```python
from build123d import *

# Parameters (mm, degrees)
BOSS_EXTRUDE1_DEPTH = 5


with BuildPart() as part:
    # Sketch1 → Boss-Extrude1 (new body)
    with BuildSketch(Plane(origin=(0, 0, 0), x_dir=(1, 0, 0), z_dir=(0, 1, 0))):
        with BuildLine():
            Line((16.51, -1.905), (16.51, 1.905))
            Line((16.51, 1.905), (12.556312158, 1.905))
            ThreePointArc((12.556312158, 1.905), (8.980256121, 8.980256121), (1.905, 12.556312158))
            Line((1.905, 12.556312158), (1.905, 16.51))
            Line((1.905, 16.51), (-1.905, 16.51))
            Line((-1.905, 16.51), (-1.905, 12.556312158))
            ThreePointArc((-1.905, 12.556312158), (-8.980256121, 8.980256121), (-12.556312158, 1.905))
            Line((-12.556312158, 1.905), (-16.51, 1.905))
            Line((-16.51, 1.905), (-16.51, -1.905))
            Line((-16.51, -1.905), (-12.556312158, -1.905))
            ThreePointArc((-12.556312158, -1.905), (-8.980256121, -8.980256121), (-1.905, -12.556312158))
            Line((-1.905, -12.556312158), (-1.905, -16.51))
            Line((-1.905, -16.51), (1.905, -16.51))
            Line((1.905, -16.51), (1.905, -12.556312158))
            ThreePointArc((1.905, -12.556312158), (8.980256121, -8.980256121), (12.556312158, -1.905))
            Line((12.556312158, -1.905), (16.51, -1.905))
        make_face()
    extrude(amount=BOSS_EXTRUDE1_DEPTH)


solid = part.part
```
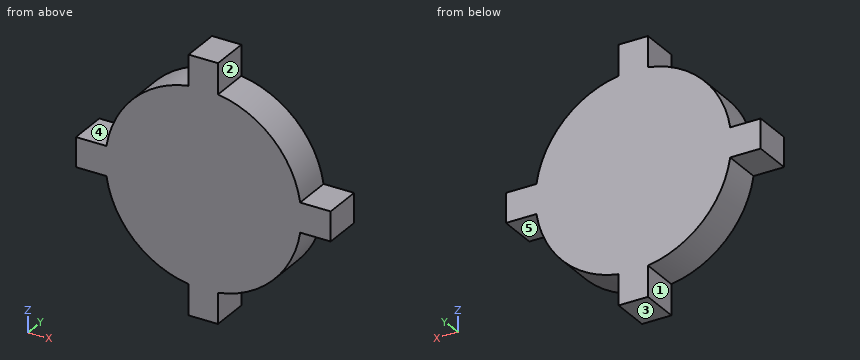
Input: part model. Units: mm. Frame: model coordinates. Face numbers are marked on the shaded views. A direction names the side the tool comes from. Give positions to 0.01 mm unless a question says otherwise; leave off trailing zeros. Loops run counter-clockwise (first coordinate to the right, second up) from the corner with the lowest first, then second, coordinate; pieces in that order, holes last.
1) Section query C-C on x = 14. Return the cut outline in (y, z) (3 decimals), and give its area (4 significant figures).
A:
outline: (0, -1.905) - (5, -1.905) - (5, 1.905) - (0, 1.905) - close
area: 19.05 mm2
2) Line query: L1, parallel to X at y = 0.95, z = 13 (3 decimals); L2, parallel to Z at x = 10.5, y = 3.8. Output: solid intervals per line, ascending.
A:
L1: x = -1.905 to 1.905
L2: z = -7.14 to 7.14
3) Section query A-A on y = 4.2. Return the cut outline in (x, z) (3 decimals).
A:
outline: (-16.51, -1.905) - (-12.556, -1.905) arc R12.7 ccw to (-1.905, -12.556) - (-1.905, -16.51) - (1.905, -16.51) - (1.905, -12.556) arc R12.7 ccw to (12.556, -1.905) - (16.51, -1.905) - (16.51, 1.905) - (12.556, 1.905) arc R12.7 ccw to (1.905, 12.556) - (1.905, 16.51) - (-1.905, 16.51) - (-1.905, 12.556) arc R12.7 ccw to (-12.556, 1.905) - (-16.51, 1.905) - close
4) Contact query for flat-ended pins moving along their axis: pin 1 (1.5 mm diameter, centred on y = 3.5, z = -8, fed in from -X); pin 2 (1.2 mm diameter, centred on x = 13.5, y = 1.5, fed in from -Z) (3 decimals); pin 3 (3 mm diameter, centred on x = 12.5, y = 0.5, fed in from -Z). Output: stop coordinate, or through.
A:
pin 1: stops at x = -10.43
pin 2: stops at z = -1.905
pin 3: stops at z = -6.35
5) Reachability of the marked faces 1, 2, 3, 4 and 5 from +Z, -Z, +X, -X, +Y, -Y: full face, straight path, thin tool, end or side. Return the list, or none.
A:
face 1: -Z, -X, +Y, -Y
face 2: +Z, +X, +Y, -Y
face 3: -Z, +X, -X, +Y, -Y
face 4: +Z, -X, +Y, -Y
face 5: -Z, +X, +Y, -Y
6) Section query B-B on z = -14. Return the cut outline in (x, y) (3 decimals).
A:
outline: (-1.905, 0) - (1.905, 0) - (1.905, 5) - (-1.905, 5) - close
